from build123d import *

# Parameters (mm, degrees)
F0_W           = 50
F0_H           = 27
F1_DEPTH       = 3
F2_D           = 3.4
F2_DEPTH       = 5
F2_CSINK_D     = 6.72
F2_CSINK_ANGLE = 90
F2_TIP         = 1.0214630523
F3_DEPTH       = 3
F0_H_2         = 3
F4_DEPTH       = 27
F5_DEPTH       = 10
F6_DEPTH       = 10
F7_W           = 30
F7_H           = 27
F8_DEPTH       = 7
F9_D           = 3.3
F9_DEPTH       = 14.1
F9_TIP         = 0.9914200214


with BuildPart() as f1:
    # F0 (on Front) → F1 (new body)
    with BuildSketch(Plane.XZ):
        with Locations((25, 16.5)):
            Rectangle(F0_W, F0_H)
    extrude(amount=-F1_DEPTH)

    # F2
    with Locations(Plane.XZ):
        with Locations((35, 26.5), (15, 26.5), (15, 6.5), (35, 6.5)):
            CounterSinkHole(F2_D / 2, F2_CSINK_D / 2, depth=F2_DEPTH, counter_sink_angle=F2_CSINK_ANGLE)
            with Locations((0, 0, -(F2_DEPTH + F2_TIP / 2))):  # 118° drill point
                Cone(0, F2_D / 2, F2_TIP, mode=Mode.SUBTRACT)

    # F3 (add): a face of the model
    f3_faces = [f1.faces().sort_by_distance(p)[0] for p in [
        (25, 1.5, 3),
    ]]
    extrude(f3_faces, amount=F3_DEPTH)

    # F0 (on Front) → F4 (join)
    with BuildSketch(Plane.XZ):
        with Locations((25, 1.5)):
            Rectangle(F0_W, F0_H_2)
    extrude(amount=F4_DEPTH)

    # F5 (add): a face of the model
    f5_faces = [f1.faces().sort_by_distance(p)[0] for p in [
        (50, 1.5, 29.5757359313),
    ]]
    extrude(f5_faces, amount=F5_DEPTH)

    # F6 (add): a face of the model
    f6_faces = [f1.faces().sort_by_distance(p)[0] for p in [
        (0, 1.5, 29.5757359313),
    ]]
    extrude(f6_faces, amount=F6_DEPTH)

    # F7 (on face) → F8 (cut)
    with BuildSketch(Plane.XY.offset(3)):
        with Locations((25, -13.5)):
            Rectangle(F7_W, F7_H)
    extrude(amount=-F8_DEPTH, mode=Mode.SUBTRACT)

    # F9
    with Locations(Plane.XY.offset(3)):
        with Locations((0, -15), (50, -15)):
            Hole(F9_D / 2, depth=F9_DEPTH)
            with Locations((0, 0, -(F9_DEPTH + F9_TIP / 2))):  # 118° drill point
                Cone(0, F9_D / 2, F9_TIP, mode=Mode.SUBTRACT)


solid = f1.part
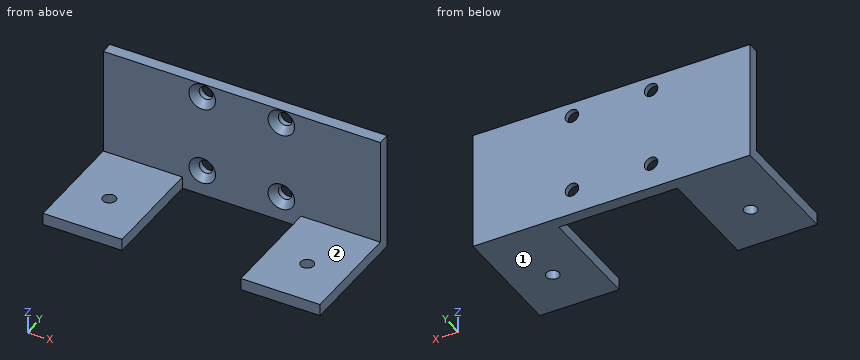
Design review of the part built by this model. Coordinates are the model's own, in mm. Face numbers are marked on the shaded views. A direction names the side the tool comes from. Round coordinates to 2 decimals unless told otherwise and drop trailing zeros. Write each loop counter-clockwise with the first axis right and the second up, starting at its lowest first coordinate (ties: lowest second). Pieces come first, ordered by that corner, then holes.
Item 1: Consider section A-A on y = -15. Give the boundary of the cut face in (x, z).
Item 2: For the marked faces 1 and 2, list the 3-axis set-ups (+Z, -Z, +X, -X, +Y, -Y) from which the entire face can be reached by the end or side of a thin tool; tool diameter is ignored.
Item 3: Consider section C-C on x = 35. Give the boundary of the cut face in (y, z), and give its area (3 significant figures).
Item 4: Wall thickness on L1, parallel to X at y = 2.2, z = 6.5; L2, parallel to Z at x = 15, y = 2.35; L3, parallel to Z at x = -1, y = -10.75: over which ranges is each line inside the solid? List them lowest first.
Item 5: Consider section B-B on x = 50. Give the boundary of the cut face in (y, z).
Item 6: For pin 1 Ø6 at (x, y) = (0.5, -7.5) entering from +Z; pin 2 Ø12 at (x, z) = (31, 10.5) entering from -Y; pin 3 Ø10 at (x, y) = (47.5, -12) entering from -Z; pin 4 Ø4.5 at (x, z) = (35, 26.5) entering from -Y, all flat-tipped, find the tip position at first contact; note any pin that passes through.
Item 7: Consider section D-D on z = 6.5. Give the boundary of the cut face in (x, y), and give its area (3 significant figures).
Check values:
1. outline: (-10, 0) - (-1.65, 0) - (-1.65, 3) - (-10, 3) - close; (1.65, 0) - (10, 0) - (10, 3) - (1.65, 3) - close; (40, 0) - (48.35, 0) - (48.35, 3) - (40, 3) - close; (51.65, 0) - (60, 0) - (60, 3) - (51.65, 3) - close
2. face 1: -Z, +X, -X, +Y, -Y
2. face 2: +Z, +X, -X, -Y
3. outline: (0, 0) - (3, 0) - (3, 4.8) - (1.66, 4.8) - (0, 3.14) - close; (0, 9.86) - (1.66, 8.2) - (3, 8.2) - (3, 24.8) - (1.66, 24.8) - (0, 23.14) - close; (0, 29.86) - (1.66, 28.2) - (3, 28.2) - (3, 30) - (0, 30) - close
3. area: 64.1 mm2
4. L1: x = -10 to 13.3, 16.7 to 33.3, 36.7 to 60
4. L2: z = 0 to 4.8, 8.2 to 24.8, 28.2 to 30
4. L3: z = 0 to 3
5. outline: (-27, 0) - (-16.65, 0) - (-16.65, 3) - (-27, 3) - close; (-13.35, 0) - (3, 0) - (3, 30) - (0, 30) - (0, 3) - (-13.35, 3) - close
6. pin 1: stops at z = 3
6. pin 2: stops at y = 0
6. pin 3: stops at z = 0
6. pin 4: stops at y = 1.11
7. outline: (-10, 0) - (11.64, 0) - (13.3, 1.66) - (13.3, 3) - (-10, 3) - close; (16.7, 1.66) - (18.36, 0) - (31.64, 0) - (33.3, 1.66) - (33.3, 3) - (16.7, 3) - close; (36.7, 1.66) - (38.36, 0) - (60, 0) - (60, 3) - (36.7, 3) - close
7. area: 184 mm2
